Check sheet for the drawn part. Datum: minimum x, y, z corner. Units: mm. Round coordinates to 2 decimals unless told otherwise and drop trailing zeros. Write each loop counter-clockwise with the first axis right and the second up, starting at its lowest first coordinate (ties: lowest second). Pieces come first, ordered by that corner, then holes. Notation, with made-up numbers: (3.25, 63) - (22.25, 63) arc R18 ccw to (22.25, 72) - close; hole circle Ø5 at (38.25, 7.25). An arc over 180 degrees is marked (long way). Answer as a JSON object with one key per item and string values.
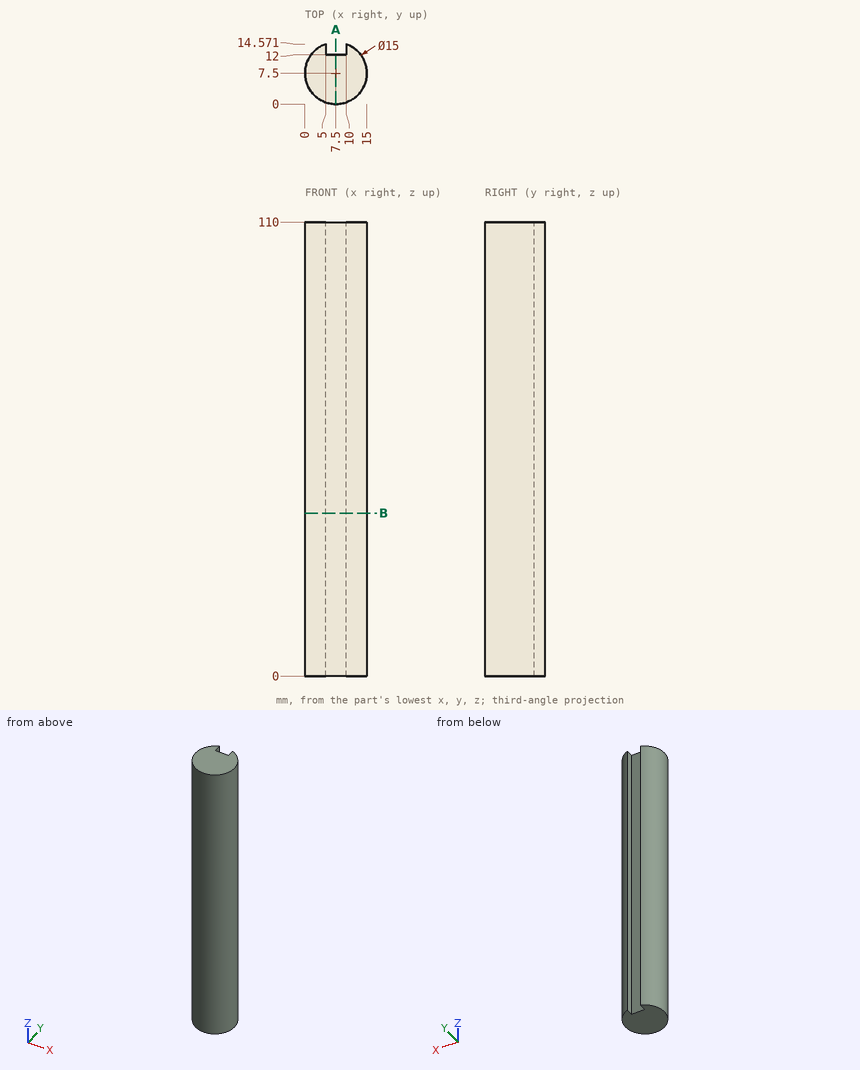
1. Go/stop test with flat-tipped pins: pin 1 (3 mm diameter, centred on y = 13.5, z = 44.5, fed in from -X); pin 2 (6 mm diameter, centred on y = 4, z = 77.5, fed in from +X); pin 3 (1.5 mm diameter, centred on y = 11.5, z = 77.5, fed in from +X); pin 4 (8 mm diameter, centred on y = 8.5, z = 92, fed in from -X). Record where each tip stops, or that it passes through.
Completed:
{"pin 1": "stops at x = 1.5", "pin 2": "stops at x = 14.98", "pin 3": "stops at x = 14.26", "pin 4": "stops at x = 0"}
2. Material ranges on probe 1 along Y at (x, z) = (7, 57.5); probe 2 along X at (y, z) = (13.75, 77); probe 3 along X at (y, z) = (6.5, 46.5), recorded low to high. Write a range as from..to.
Completed:
{"probe 1": "y = 0.02..12", "probe 2": "x = 3.35..5, 10..11.65", "probe 3": "x = 0.07..14.93"}
3. Cross-section at A-A (x = 7.5). Record the boundary of the cut face in (y, z).
Completed:
{"outline": "(0, 0) - (12, 0) - (12, 110) - (0, 110) - close"}
4. Cross-section at B-B (z = 39.5). Record the boundary of the cut face in (x, y), plus the area to 3 significant figures.
Completed:
{"outline": "(5, 12) - (5, 14.57) arc R7.5 ccw (long way) to (10, 14.57) - (10, 12) - close", "area": "162 mm^2"}
